Can you work these out from the model? Positions are in its coordinate system, mm. A direction names the side the tool comes from. Give positions to 0.01 mm unless a question says otherwise; leave off trailing zeros. Loops run counter-clockwise (first coordinate to the right, second up) from the corner with the lowest first, then second, coordinate; pieces in that order, holes last. Notation, with made-up numbers: (56.5, 12) - (108.5, 12) arc R28 cw to (108.5, 38) - close; hole circle Ø7 at (7, 18.25). An arc over 180 degrees is marked (long way). Use a Markdown table: item, result. Add a question column.
```python
from build123d import *


with BuildPart() as f1:
    # F0 (on Front) → F1 (revolve)
    with BuildSketch(Plane.XZ):
        with BuildLine():
            Line((-19.466886, 0), (0, 0))
            Line((0, 0), (0, 97.4))
            ThreePointArc((0, 97.4), (0.279718, 97.781487), (0.727661, 97.629431))
            Line((0.727661, 97.629431), (0.818289, 97.5))
            Line((0.818289, 97.5), (11.6, 97.5))
            Line((11.6, 97.5), (11.6, 111.944042))
            Line((11.6, 111.944042), (-19.466886, 111.944042))
            Line((-19.466886, 111.944042), (-19.466886, 0))
        make_face()
    revolve(axis=Axis((-9.733443, 0, 0), (-1, 0, 0)))


solid = f1.part
```
1. Suppose I cut it at C-C (x = 6). List the corners of the cut face in (y, z) for me.
2. On a 3-axis mill with a long thin cutter (end or side, diameter ignored), from which of +Z, -Z, +X, -X, +Y, -Y can I reach the whole of each face in a straight line? I mean faces 4 (the face through (11.6, 92, 34)), 5 (the face through (0, 1, 1)). Say none if no direction works.
3. Suppose I cut it at A-A (z = 0). List the corners of the cut face in (x, y) for me, and give its area (3 significant figures).
4. Will these pins go through, and if not, where does the flat tip stop? P1, Ø3, axis at x = -1.5, z = -80, coming from the -Y side; P2, Ø1, axis at x = -11, y = 63, coming from the -Z side; P3, Ø2, axis at x = 5, z = 86.5, coming from the -Y side; P4, Ø10, axis at y = 85, z = -75.5, coming from the -X side.
5. Please list where these lines run through material, in increasing order: line 1 along Y through (x, z) = (9, 0); line 2 along X through (y, z) = (63.5, 15.5); line 3 along Z through (x, y) = (9.5, -52.5). Write a range as [from, to].
6. If we mould it in two halves opening along Y, with no side actions, what happens to faces 1 (the face through (-19.467, 2, -2)), 2 (the face through (-4.15, 110.99, -14.57)), 3 (the face through (6.28, -59.33, -77.37))? For each: released by +Y, released by -Y, zero draft, split by the parting line, or undercut.
Results below:
| question | item | result |
|---|---|---|
| 1 | outline | circle Ø223.89 at (0, 0); hole circle Ø195 at (0, 0) |
| 2 | face 4 | +Z, -Z, +X, +Y, -Y |
| 2 | face 5 | +X |
| 3 | outline | (-19.47, -111.94) - (11.6, -111.94) - (11.6, -97.5) - (0.82, -97.5) - (0.73, -97.63) arc R0.4 cw to (0, -97.4) - (0, 97.4) arc R0.4 cw to (0.73, 97.63) - (0.82, 97.5) - (11.6, 97.5) - (11.6, 111.94) - (-19.47, 111.94) - close |
| 3 | area | 4,690 mm² |
| 4 | P1 | y = -79.81 |
| 4 | P2 | z = -92.87 |
| 4 | P3 | y = -72.26 |
| 4 | P4 | x = -19.47 |
| 5 | line 1 | [-111.94, -97.5], [97.5, 111.94] |
| 5 | line 2 | [-19.47, 0] |
| 5 | line 3 | [-98.87, -82.16], [82.16, 98.87] |
| 6 | face 1 | zero draft |
| 6 | face 2 | split by the parting line |
| 6 | face 3 | undercut |
